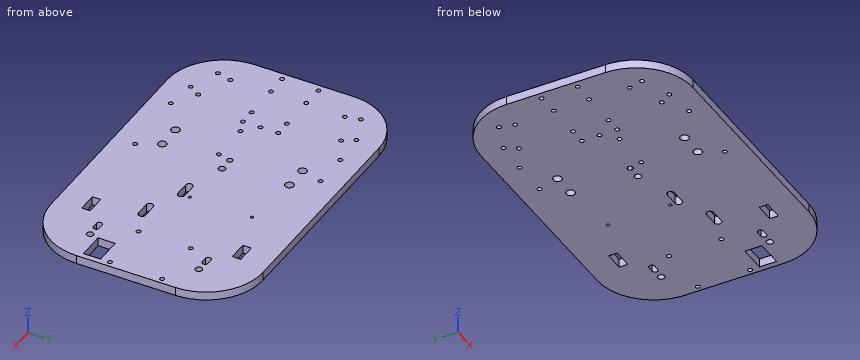
from build123d import *

# Parameters (mm, degrees)
ESBO_O1_R                   = 1.55
ESBO_O1_R_2                 = 2.4
ESBO_O1_R_3                 = 1.05
ESBO_O1_W                   = 18.9
ESBO_O1_H                   = 12.1
ESBO_O1_W_2                 = 13.55
ESBO_O1_H_2                 = 6.05
RESSALTO_EXTRUS_O1_DEPTH    = 6
CORTE_EXTRUS_O1_START       = -6
CORTE_EXTRUS_O1_OUTLINE_R   = 2.999999997
CORTE_EXTRUS_O1_OUTLINE_R_2 = 2.55
CORTE_EXTRUS_O1_OUTLINE_R_3 = 1.55
CORTE_EXTRUS_O1_DEPTH       = 6
RESSALTO_EXTRUS_O2_DEPTH    = 6
CORTE_EXTRUS_O2_DEPTH       = 6
ESBO_O5_R                   = 2.05
CORTE_EXTRUS_O3_DEPTH       = 6
RESSALTO_EXTRUS_O3_DEPTH    = 6
ESBO_O8_W                   = 50
ESBO_O8_H                   = 9.999552213
ESBO_O8_H_2                 = 10.000447787
RESSALTO_EXTRUS_O4_DEPTH    = 6
ESBO_O9_R                   = 3.05
CORTE_EXTRUS_O4_DEPTH       = 6
ESBO_O10_R                  = 1.05
RESSALTO_EXTRUS_O5_DEPTH    = 6
ESBO_O11_R                  = 1.05
CORTE_EXTRUS_O5_DEPTH       = 6


# Read off the part's stored shape, not the designer's step: Corte-extrusão1
with BuildPart() as part:
    # Esboço1 → Ressalto-extrusão1 (new body)
    with BuildSketch(Plane.XY):
        with BuildLine():
            Line((-57.793944221, 57.049862318), (92.206055779, 57.049862318))
            ThreePointArc((92.206055779, 57.049862318), (120.490327027, 45.334133565), (132.206055779, 17.049862318))
            Line((132.206055779, 17.049862318), (132.206055779, -52.950137682))
            ThreePointArc((132.206055779, -52.950137682), (120.490327027, -81.234408929), (92.206055779, -92.950137682))
            Line((92.206055779, -92.950137682), (-57.793944221, -92.950137682))
            ThreePointArc((-57.793944221, -92.950137682), (-86.078215468, -81.234408929), (-97.793944221, -52.950137682))
            Line((-97.793944221, -52.950137682), (-97.793944221, 17.049862318))
            ThreePointArc((-97.793944221, 17.049862318), (-86.078215468, 45.334133565), (-57.793944221, 57.049862318))
        make_face()
        with Locations((91.206055779, 5.549862318)):
            Circle(ESBO_O1_R, mode=Mode.SUBTRACT)
        with Locations((-78.899831671, -68.557958731)):
            Circle(ESBO_O1_R, mode=Mode.SUBTRACT)
        with Locations((91.206055779, -31.450137682)):
            Circle(ESBO_O1_R, mode=Mode.SUBTRACT)
        with Locations((-53.299831671, -68.557958731)):
            Circle(ESBO_O1_R, mode=Mode.SUBTRACT)
        with Locations((128.206055779, -31.450137682)):
            Circle(ESBO_O1_R, mode=Mode.SUBTRACT)
        with Locations((-77.788996209, -5.451057304)):
            Circle(ESBO_O1_R, mode=Mode.SUBTRACT)
        with Locations((11.222430841, -77.710137682)):
            Circle(ESBO_O1_R, mode=Mode.SUBTRACT)
        with Locations((-37.037569159, -78.980137682)):
            Circle(ESBO_O1_R, mode=Mode.SUBTRACT)
        with Locations((-31.957569159, -26.910137682)):
            Circle(ESBO_O1_R, mode=Mode.SUBTRACT)
        with Locations((-4.017569159, -26.910137682)):
            Circle(ESBO_O1_R, mode=Mode.SUBTRACT)
        with Locations((128.206055779, 5.549862318)):
            Circle(ESBO_O1_R, mode=Mode.SUBTRACT)
        with Locations((-92.793944221, -30.750137682)):
            Circle(ESBO_O1_R, mode=Mode.SUBTRACT)
        with Locations((-92.793944221, -5.150137682)):
            Circle(ESBO_O1_R, mode=Mode.SUBTRACT)
        with Locations((-76.401765269, 22.555749768)):
            Circle(ESBO_O1_R, mode=Mode.SUBTRACT)
        with Locations((-52.788996209, -5.451057304)):
            Circle(ESBO_O1_R, mode=Mode.SUBTRACT)
        with Locations((-52.788996209, -30.451057304)):
            Circle(ESBO_O1_R, mode=Mode.SUBTRACT)
        with Locations((-77.788996209, -30.451057304)):
            Circle(ESBO_O1_R, mode=Mode.SUBTRACT)
        with Locations((-78.899831671, 32.657683367)):
            Circle(ESBO_O1_R, mode=Mode.SUBTRACT)
        with Locations((-53.299831671, 32.657683367)):
            Circle(ESBO_O1_R, mode=Mode.SUBTRACT)
        with Locations((-58.299831671, 40.657683367)):
            Circle(ESBO_O1_R, mode=Mode.SUBTRACT)
        with Locations((-58.299831671, -76.557958731)):
            Circle(ESBO_O1_R, mode=Mode.SUBTRACT)
        with Locations((-76.401765269, -58.456025132)):
            Circle(ESBO_O1_R, mode=Mode.SUBTRACT)
        with Locations((-35.15079847, 31.606716567)):
            Circle(ESBO_O1_R, mode=Mode.SUBTRACT)
        with Locations((-9.55079847, 31.606716567)):
            Circle(ESBO_O1_R, mode=Mode.SUBTRACT)
        with Locations((108.206055779, -56.450137682)):
            Circle(ESBO_O1_R_2, mode=Mode.SUBTRACT)
        with Locations((108.206055779, 20.549862318)):
            Circle(ESBO_O1_R_2, mode=Mode.SUBTRACT)
        with Locations((44.206055779, -19.950137682)):
            Circle(ESBO_O1_R_3, mode=Mode.SUBTRACT)
        with Locations((8.206055779, -17.950137682)):
            Circle(ESBO_O1_R_2, mode=Mode.SUBTRACT)
        with Locations((44.206055779, 24.049862318)):
            Circle(ESBO_O1_R_3, mode=Mode.SUBTRACT)
        with Locations((-41.520254265, -30.451057304)):
            Circle(ESBO_O1_R, mode=Mode.SUBTRACT)
        with Locations((-41.520254265, -17.951057304)):
            Circle(ESBO_O1_R, mode=Mode.SUBTRACT)
        with Locations((-41.520254265, -5.451057304)):
            Circle(ESBO_O1_R, mode=Mode.SUBTRACT)
        with BuildLine():
            Line((74.102198496, -40.878145103), (64.102198496, -40.878145103))
            ThreePointArc((64.102198496, -40.878145103), (61.602198496, -38.378145103), (64.102198496, -35.878145103))
            Line((64.102198496, -35.878145103), (74.102198496, -35.878145103))
            ThreePointArc((74.102198496, -35.878145103), (76.602198496, -38.378145103), (74.102198496, -40.878145103))
        make_face(mode=Mode.SUBTRACT)
        with BuildLine():
            Line((96.206055779, 22.549862318), (100.206055779, 22.549862318))
            ThreePointArc((100.206055779, 22.549862318), (102.206055779, 20.549862318), (100.206055779, 18.549862318))
            Line((100.206055779, 18.549862318), (96.206055779, 18.549862318))
            ThreePointArc((96.206055779, 18.549862318), (94.206055779, 20.549862318), (96.206055779, 22.549862318))
        make_face(mode=Mode.SUBTRACT)
        with BuildLine():
            Line((96.206055779, -54.450137682), (100.206055779, -54.450137682))
            ThreePointArc((100.206055779, -54.450137682), (102.206055779, -56.450137682), (100.206055779, -58.450137682))
            Line((100.206055779, -58.450137682), (96.206055779, -58.450137682))
            ThreePointArc((96.206055779, -58.450137682), (94.206055779, -56.450137682), (96.206055779, -54.450137682))
        make_face(mode=Mode.SUBTRACT)
        with Locations((118.766338719, -44.142882399)):
            Rectangle(ESBO_O1_W, ESBO_O1_H, mode=Mode.SUBTRACT)
        with Locations((79.761339118, 35.337517738)):
            Rectangle(ESBO_O1_W_2, ESBO_O1_H_2, mode=Mode.SUBTRACT)
        with Locations((79.761339118, -71.237793102)):
            Rectangle(ESBO_O1_W_2, ESBO_O1_H_2, mode=Mode.SUBTRACT)
    extrude(amount=RESSALTO_EXTRUS_O1_DEPTH)

    # Corte-extrusão1 outline → Corte-extrusão1 (cut)
    with BuildSketch(Plane.XY.offset(6).offset(CORTE_EXTRUS_O1_START)):
        with Locations((-17.788996212, -62.950585469)):
            Circle(CORTE_EXTRUS_O1_OUTLINE_R)
        with Locations((7.211003788, -62.950585469)):
            Circle(CORTE_EXTRUS_O1_OUTLINE_R)
        with Locations((-17.788996212, 27.049414531)):
            Circle(CORTE_EXTRUS_O1_OUTLINE_R)
        with Locations((7.211003788, 27.049414531)):
            Circle(CORTE_EXTRUS_O1_OUTLINE_R)
        with Locations((0.411003785, -17.950228357)):
            Circle(CORTE_EXTRUS_O1_OUTLINE_R_2)
        with Locations((-35.15079847, 42.049862318)):
            Circle(CORTE_EXTRUS_O1_OUTLINE_R_3)
        with Locations((-9.55079847, 42.049862318)):
            Circle(CORTE_EXTRUS_O1_OUTLINE_R_3)
    extrude(amount=CORTE_EXTRUS_O1_DEPTH, mode=Mode.SUBTRACT)

    # Esboço3 → Ressalto-extrusão2 (add)
    with BuildSketch(Plane.XY.offset(6)):
        Polygon((-14.016641423, 28.740365826), (0, 28.740365826), (0, 35.849208008), (-40.162042527, 35.849208008), (-40.162042527, 28.740365826), (-25.883056006, 28.740365826), (-25.883056006, 31.312651868), (-14.016641423, 31.312651868), align=None)
    extrude(amount=-RESSALTO_EXTRUS_O2_DEPTH)

    # Esboço4 → Corte-extrusão2 (cut)
    with BuildSketch(Plane.XY.offset(6)):
        with BuildLine():
            Line((44.103196828, -24.450137682), (34.103196828, -24.450137682))
            ThreePointArc((34.103196828, -24.450137682), (31.603196828, -26.950137682), (34.103196828, -29.450137682))
            Line((34.103196828, -29.450137682), (44.103196828, -29.450137682))
            ThreePointArc((44.103196828, -29.450137682), (46.603196828, -26.950137682), (44.103196828, -24.450137682))
        make_face()
    extrude(amount=-CORTE_EXTRUS_O2_DEPTH, mode=Mode.SUBTRACT)

    # Esboço5 → Corte-extrusão3 (cut)
    with BuildSketch(Plane.XY.offset(6)):
        with Locations((-1.793944221, -17.950137682)):
            Circle(ESBO_O5_R)
    extrude(amount=-CORTE_EXTRUS_O3_DEPTH, mode=Mode.SUBTRACT)

    # Esboço6 → Ressalto-extrusão3 (add)
    with BuildSketch(Plane.XY.offset(6)):
        with BuildLine():
            ThreePointArc((0.256055779, -17.950137682), (-0.344375319, -19.399706583), (-1.793944221, -20.000137682))
            Line((-1.793944221, -20.000137682), (-1.793944221, -22.624881404))
            Line((-1.793944221, -22.624881404), (3.749048886, -22.624881404))
            Line((3.749048886, -22.624881404), (3.749048886, -13.412148233))
            Line((3.749048886, -13.412148233), (-1.793944221, -13.412148233))
            Line((-1.793944221, -13.412148233), (-1.793944221, -15.900137682))
            ThreePointArc((-1.793944221, -15.900137682), (-0.344375319, -16.500568781), (0.256055779, -17.950137682))
        make_face()
    extrude(amount=-RESSALTO_EXTRUS_O3_DEPTH)

    # Esboço8 → Ressalto-extrusão4 (add)
    with BuildSketch(Plane.XY.offset(6)):
        with Locations((-5.288996218, -62.950361576)):
            Rectangle(ESBO_O8_W, ESBO_O8_H)
        with Locations((-5.288996218, 27.049638425)):
            Rectangle(ESBO_O8_W, ESBO_O8_H_2)
    extrude(amount=-RESSALTO_EXTRUS_O4_DEPTH)

    # Esboço9 → Corte-extrusão4 (cut)
    with BuildSketch(Plane.XY.offset(6)):
        with Locations((-13.788996218, -62.950361575)):
            Circle(ESBO_O9_R)
        with Locations((3.211003782, -62.950361575)):
            Circle(ESBO_O9_R)
        with Locations((3.211003782, 27.050086211)):
            Circle(ESBO_O9_R)
        with Locations((-13.788996218, 27.050086211)):
            Circle(ESBO_O9_R)
    extrude(amount=-CORTE_EXTRUS_O4_DEPTH, mode=Mode.SUBTRACT)

    # Esboço10 → Ressalto-extrusão5 (add)
    with BuildSketch(Plane(origin=(0, 0, 0), x_dir=(-1, 0, 0), z_dir=(0, 0, -1))):
        with Locations((-44.206055779, -19.950137682)):
            Circle(ESBO_O10_R)
        with Locations((-44.206055779, 24.049862318)):
            Circle(ESBO_O10_R)
    extrude(amount=-RESSALTO_EXTRUS_O5_DEPTH)

    # Esboço11 → Corte-extrusão5 (cut)
    with BuildSketch(Plane(origin=(0, 0, 0), x_dir=(-1, 0, 0), z_dir=(0, 0, -1))):
        with Locations((-44.206055779, 23.049862318)):
            Circle(ESBO_O11_R)
        with Locations((-44.206055779, -20.950137682)):
            Circle(ESBO_O11_R)
    extrude(amount=-CORTE_EXTRUS_O5_DEPTH, mode=Mode.SUBTRACT)


solid = part.part
Here's how the part is built. I have some questions about the finished solid (model axes, mm). Round coordinates to 2 decimals unless told otherwise and drop trailing zeros. Write each loop counter-clockwise with the first axis right and the second up, starting at its lowest first coordinate (ties: lowest second). Pieces come first, ordered by that corner, then holes. Notation, with made-up numbers: (74, -15.5) -> (99, -15.5) arc R22 cw to (99, -5.5) -> close; hole circle Ø1 at (37.25, 39). An arc over 180 degrees is marked (long way). One line per item, written item: value.
1) If I drill on line 1 (Y direction, x = 74, z = 1.8); line 2 (Y direction, x = 72, z = 0.7); line 3 (Y direction, x = -16, z = 4.75), over which ranges is the centre line in solid material (lowest first)? Write a range as [from, to].
Filled sheet:
line 1: y = [-92.95, -74.26], [-68.21, -40.88], [-35.88, 32.31], [38.36, 57.05]
line 2: y = [-92.95, -40.88], [-35.88, 57.05]
line 3: y = [-92.95, -65.05], [-60.85, 24.95], [29.15, 57.05]
2) Suppose I cut it at B-B on z = 2.2. Give the number of separate pieces and of enclosed holes in the cut face, plus the area to 3 significant figures.
Filled sheet:
separate pieces: 1
enclosed holes: 44
area: 32,100 mm2
3) Suppose I cut it at A-A on y = -47. List the corners of the cut face in (x, z) for me.
Filled sheet:
outline: (-97.79, 0) -> (109.32, 0) -> (109.32, 6) -> (-97.79, 6) -> close; (128.22, 0) -> (132.21, 0) -> (132.21, 6) -> (128.22, 6) -> close
4) I'm going to push flat-ended pins straight in: pin 1 Ø2 at (y, z) = (27.5, 1) entering from +X; pin 2 Ø2 at (y, z) = (32, 1) entering from +X; pin 3 Ø3 at (y, z) = (-70.5, 2) entering from +X; pin 4 Ø1.9 at (x, y) = (44.21, 23.05) entering from +Z. Where does each tip first touch, or does it pass through?
Filled sheet:
pin 1: stops at x = 131.07
pin 2: stops at x = 129.69
pin 3: stops at x = 128.84
pin 4: passes through
